```python
from build123d import *

# Parameters (mm, degrees)
EXTRUDE_1_DEPTH     = 6.5
FILLET_1_R          = 2
FILLET_2_R          = 1.5
SKETCH_2_W          = 6
SKETCH_2_H          = 0.875
CUT_EXTRUDE_1_DEPTH = 10
FILLET_4_R          = 1
FILLET_5_R          = 0.1
FILLET_6_R          = 0.1
SKETCH_3_W          = 2.25
SKETCH_3_H          = 1.5
CUT_EXTRUDE_2_DEPTH = 10


with BuildPart() as part:
    # Эскиз1 → Бобышка-Вытянуть1 (new body)
    with BuildSketch(Plane(origin=(0, 0, 0), x_dir=(1, 0, 0), z_dir=(0, 1, 0))):
        Polygon((-22.702464419, 0), (-21.702464419, 0), (-21.702464419, 8), (-13.702464419, 8), (-13.702464419, 9), (-22.702464419, 9), align=None)
    extrude(amount=EXTRUDE_1_DEPTH)

    # Скругление1
    fillet_1_edges = [part.edges().sort_by_distance(p)[0] for p in [
        (-22.702464419, 3.25, -9),
    ]]
    fillet(fillet_1_edges, radius=FILLET_1_R)

    # Скругление2
    fillet_2_edges = [part.edges().sort_by_distance(p)[0] for p in [
        (-21.702464419, 3.25, -8),
    ]]
    fillet(fillet_2_edges, radius=FILLET_2_R)

    # Эскиз2 → Вырез-Вытянуть1 (cut, through all)
    with BuildSketch(Plane(origin=(0, 0, -9), x_dir=(-1, 0, 0), z_dir=(0, 0, -1))):
        with Locations((16.702464419, 0.4375)):
            Rectangle(SKETCH_2_W, SKETCH_2_H)
        with Locations((16.702464419, 6.0625)):
            Rectangle(SKETCH_2_W, SKETCH_2_H)
    extrude(amount=-CUT_EXTRUDE_1_DEPTH, mode=Mode.SUBTRACT)

    # Скругление4
    fillet_4_edges = [part.edges().sort_by_distance(p)[0] for p in [
        (-13.702464419, 0.875, -8.5),
        (-13.702464419, 5.625, -8.5),
    ]]
    fillet(fillet_4_edges, radius=FILLET_4_R)

    # Скругление5
    fillet_5_edges = [part.edges().sort_by_distance(p)[0] for p in [
        (-19.702464419, 0, -8.5),
        (-19.702464419, 6.5, -8.5),
    ]]
    fillet(fillet_5_edges, radius=FILLET_5_R)

    # Скругление6
    fillet_6_edges = [part.edges().sort_by_distance(p)[0] for p in [
        (-19.702464419, 0.875, -8.5),
        (-19.702464419, 5.625, -8.5),
    ]]
    fillet(fillet_6_edges, radius=FILLET_6_R)

    # Эскиз3 → Вырез-Вытянуть2 (cut, through all)
    with BuildSketch(Plane(origin=(0, 0, -9), x_dir=(-1, 0, 0), z_dir=(0, 0, -1))):
        with Locations((16.273003047, 3.25)):
            Rectangle(SKETCH_3_W, SKETCH_3_H)
    extrude(amount=-CUT_EXTRUDE_2_DEPTH, mode=Mode.SUBTRACT)


solid = part.part
```
Here's how the part is built. I have some questions about the finished solid (model axes, mm). A direction names the side the tool comes from. Coordinates: 2 decimals unless noted, no trailing zeros. Order: outer loops, then holes, each group sorted by start corner. A loop starts at its lowest first (then second) coordinate and runs counter-clockwise, first axis right, second up. Notation, with made-up numbers: (-26, -37) - (-8, -37) arc R21 ccw to (-8, -21) - close; hole circle Ø5 at (-29.75, 6). An arc over 180 degrees is marked (long way). One line per question, with ' | ' between items. Start each with the question number.
1. I'm going to push flat-ended pins straight in: pin 1 Ø0.5 at (x, z) = (-16.5, -8.5) entering from +Y (3 decimals); pin 2 Ø1.1 at (x, z) = (-16.5, -8.5) entering from -Y (3 decimals); pin 3 Ø2 at (x, y) = (-19, 3) entering from +Z. Where does each tip first touch, or does it pass through?
2. Which directions (+Z, -Z, +X, -X, +Y, -Y) give clear straight access to the entire face, cutting with the end or side of a thin tool? Please do faces 1 (the flat face through (-17.1, 0.875, -8.5)), 2 (the flat face through (-18, 3, -9)), 3 (the flat face through (-15.148, 3.2, -8.5)), 4 (the flat face through (-18, 3, -8)), 5 (the flat face through (-17.1, 5.625, -8.5)).
3. If we section it at D-D (z = -3): Write out the boundary of the cut face in (x, y).
4. If we section it at A-A (y = 3): Write out the boundary of the cut face in (x, z).
5. If we section it at B-B (x = -17): Write out the boundary of the cut face in (y, z) (3 decimals).
6. Please list where these lines run through material, in increasing order: line 1 along Y through (x, z) = (-14.75, -8.25) (3 decimals); line 2 along X through (y, z) = (5.5, -1); line 3 along Z through (x, y) = (-15.25, 4.5). Write a range as [from, to].
7. If we section it at C-C (y = 0.5): Write out the boundary of the cut face in (x, z), and give its area (3 significant figures).
8. If we mould it in two halves opening along Y, with no side actions, what happens to faces 6 (the flat face through (-17.398, 3.2, -8.5)), 7 (the flat face through (-22, 0, -6)), 8 (the cylindrical face through (-21.251, 3.296, -7.572)), 9 (the flat face through (-16.3, 4, -8.5))? For each: released by +Y, released by -Y, zero draft, split by the parting line, or undercut.
Model answer:
1) pin 1: stops at y = 5.625 | pin 2: stops at y = 0.875 | pin 3: stops at z = -8
2) face 1: +Z, -Z, +X, -Y | face 2: -Z, +X, -X, +Y, -Y | face 3: +Z, -Z | face 4: +Z, +X, +Y, -Y | face 5: +Z, -Z, +X, +Y
3) outline: (-22.7, 0) - (-21.7, 0) - (-21.7, 6.5) - (-22.7, 6.5) - close
4) outline: (-22.7, -7) arc R2 ccw to (-20.7, -9) - (-17.4, -9) - (-17.4, -8) - (-20.2, -8) arc R1.5 cw to (-21.7, -6.5) - (-21.7, 0) - (-22.7, 0) - close; (-15.15, -9) - (-13.7, -9) - (-13.7, -8) - (-15.15, -8) - close
5) outline: (0.875, -9) - (2.5, -9) - (2.5, -8) - (0.875, -8) - close; (4, -9) - (5.625, -9) - (5.625, -8) - (4, -8) - close
6) line 1: y = [0.875, 5.625] | line 2: x = [-22.7, -21.7] | line 3: z = [-9, -8]
7) outline: (-22.7, -7) arc R2 ccw to (-20.7, -9) - (-19.7, -9) - (-19.7, -8) - (-20.2, -8) arc R1.5 cw to (-21.7, -6.5) - (-21.7, 0) - (-22.7, 0) - close | area: 10.6 mm²
8) face 6: undercut | face 7: released by -Y | face 8: zero draft | face 9: undercut
